```python
from build123d import *

# Parameters (mm, degrees)
SKETCH2_R           = 1.75
BOSS_EXTRUDE1_DEPTH = 10
SKETCH3_W           = 7.5
SKETCH3_H           = 3
BOSS_EXTRUDE2_DEPTH = 5
SKETCH4_W           = 15
SKETCH4_H           = 2
BOSS_EXTRUDE3_DEPTH = 20
SKETCH5_W           = 12
SKETCH5_H           = 17
CUT_EXTRUDE1_DEPTH  = 1
CUT_EXTRUDE2_DEPTH  = 12
BOSS_EXTRUDE4_DEPTH = 10
SKETCH8_W           = 7.5
SKETCH8_H           = 2
BOSS_EXTRUDE5_DEPTH = 11
BOSS_EXTRUDE6_START = -7.5
SKETCH9_R           = 2
BOSS_EXTRUDE6_DEPTH = 7.5
SKETCH10_R          = 1
CUT_EXTRUDE3_DEPTH  = 31.340772897


with BuildPart() as part:
    # Sketch2 → Boss-Extrude1 (new body)
    with BuildSketch(Plane(origin=(0, 0, 0), x_dir=(0, 0, -1), z_dir=(1, 0, 0))):
        Circle(SKETCH2_R)
    extrude(amount=BOSS_EXTRUDE1_DEPTH)

    # Sketch3 → Boss-Extrude2 (add)
    with BuildSketch(Plane.XY):
        with Locations((5, 0)):
            Rectangle(SKETCH3_W, SKETCH3_H)
    extrude(amount=BOSS_EXTRUDE2_DEPTH)

    # Sketch4 → Boss-Extrude3 (add)
    with BuildSketch(Plane.XY.offset(5)):
        with Locations((5, -0.5)):
            Rectangle(SKETCH4_W, SKETCH4_H)
    extrude(amount=BOSS_EXTRUDE3_DEPTH)

    # Sketch5 → Cut-Extrude1 (cut)
    with BuildSketch(Plane(origin=(0, 0.5, 0), x_dir=(1, 0, 0), z_dir=(0, 1, 0))):
        with Locations((5, -15)):
            Rectangle(SKETCH5_W, SKETCH5_H)
    extrude(amount=-CUT_EXTRUDE1_DEPTH, mode=Mode.SUBTRACT)

    # Sketch6 → Cut-Extrude2 (cut)
    with BuildSketch(Plane.ZY.offset(-11)):
        Polygon((23.5, -0.5), (25, 0.5), (23.5, 0.5), align=None)
    extrude(amount=CUT_EXTRUDE2_DEPTH, mode=Mode.SUBTRACT)

    # Sketch7 → Boss-Extrude4 (add)
    with BuildSketch(Plane(origin=(0, 0.5, 0), x_dir=(1, 0, 0), z_dir=(0, 1, 0))):
        Polygon((-2.5, -5), (12.5, -5), (12.5, -8), (11, -8), (11, -6.5), (-1, -6.5), (-1, -8), (-2.5, -8), align=None)
    extrude(amount=BOSS_EXTRUDE4_DEPTH)

    # Sketch8 → Boss-Extrude5 (add)
    with BuildSketch(Plane(origin=(0, 0, 0), x_dir=(1, 0, 0), z_dir=(0, 1, 0))):
        with Locations((5, 0.098612181)):
            Rectangle(SKETCH8_W, SKETCH8_H)
    extrude(amount=BOSS_EXTRUDE5_DEPTH)

    # Sketch9 → Boss-Extrude6 (add)
    with BuildSketch(Plane.ZY.offset(-1.25).offset(BOSS_EXTRUDE6_START)):
        with Locations((-0.098612181, 11)):
            Circle(SKETCH9_R)
    extrude(amount=BOSS_EXTRUDE6_DEPTH)

    # Sketch10 → Cut-Extrude3 (cut, through all)
    with BuildSketch(Plane.ZY.offset(-1.25)):
        with Locations((-0.098612181, 11)):
            Circle(SKETCH10_R)
    extrude(amount=-CUT_EXTRUDE3_DEPTH, mode=Mode.SUBTRACT)


solid = part.part
```
For this review, take the finished solid that the model builds, in its own axes (mm). A direction names the side the tool comes from. Coordinates: 2 decimals unless noted, no trailing zeros. Order: outer loops, then holes, each group sorted by start corner. A loop starts at its lowest first (then second) coordinate and runs counter-clockwise, first axis right, second up. Notation, with made-up numbers: (72.5, 71) -> (82.5, 71) arc R24 ccw to (82.5, 106) -> close; hole circle Ø9 at (48, 17.5). An arc over 180 degrees is marked (long way). Use CSV: the item, a comma, the result in double quotes. Start each with the question number.
Item 1: We need section A-A, the plane y = 8. Give the boundary of the cut face in (x, z), then the cut area to 3 significant figures.
Item 2: We need section B-B, the plane z = 8.75. Give the boundary of the cut face in (x, y), then the cut area to 3 significant figures.
Item 3: Wall thickness on probe 1 along X at (y, z) = (-0.25, 21); probe 2 along Z at (x, y) = (1.5, 1.75); probe 3 along X at (y, z) = (4, 0.5): over which ranges is each line inside the solid? List them lowest first.
Item 4: We need section D-D, the plane z = 0. Give the boundary of the cut face in (x, y), then the cut area to 3 significant figures.
Item 5: Draft analysis for pull direction X (two halves, no side actions). For faces 1 (the face through (5.084, -0.007, 24.24)), 2 (the face through (8.75, 7, 0)), 3 (the face through (0, 0, 0)), state which applies: pulls with the +X half, pulls with the -X half, needs draft (parallel to the pull), parting line crosses it, or undercut.
Item 6: Insertion check: pin 1 (0.8 mm diameter, centred on x = 12, y = 4.5, fed in from +Z); pin 2 (4.5 mm diameter, centred on y = 8.5, z = -0.5, fed in from +X); pin 3 (4 mm diameter, centred on y = 2, z = 2.5, fed in from -X); pin 4 (3.5 mm diameter, centred on y = 3, z = 19, fed in from -X). Each pin has a flat end and moves straight along its axis. Give the tip position at first contact, or say it passes through.
Item 7: For faces 4 (the face through (5, 5, -1.099)), 5 (the face through (11, 0, 12)), 6 (the face through (12, 0.5, 16)), list the 3-axis set-ups (+Z, -Z, +X, -X, +Y, -Y) from which the entire face can be reached by the end or side of a thin tool; tool diameter is ignored.
Item 8: We need section C-C, the plane x = 3. Give the boundary of the cut face in (y, z), then the cut area to 3 significant figures.
Derived:
1,outline,"(-2.5, 5) -> (12.5, 5) -> (12.5, 8) -> (11, 8) -> (11, 6.5) -> (-1, 6.5) -> (-1, 8) -> (-2.5, 8) -> close; (1.25, -1.1) -> (8.75, -1.1) -> (8.75, 0.9) -> (1.25, 0.9) -> close"
1,area,"42.0 mm^2"
2,outline,"(-2.5, -1.5) -> (12.5, -1.5) -> (12.5, 0.5) -> (11, 0.5) -> (11, -0.5) -> (-1, -0.5) -> (-1, 0.5) -> (-2.5, 0.5) -> close"
2,area,"18.0 mm^2"
3,probe 1,"x = -2.5 to -1, 11 to 12.5"
3,probe 2,"z = -1.1 to 0.9, 5 to 6.5"
3,probe 3,"x = 1.25 to 8.75"
4,outline,"(0, -1.75) -> (10, -1.75) -> (10, 1.75) -> (8.75, 1.75) -> (8.75, 10) -> (1.25, 10) -> (1.25, 1.75) -> (0, 1.75) -> close; (1.25, 12) -> (8.75, 12) -> (8.75, 13) -> (1.25, 13) -> close"
4,area,"104 mm^2"
5,face 1,"undercut"
5,face 2,"pulls with the +X half"
5,face 3,"pulls with the -X half"
6,pin 1,"stops at z = 8"
6,pin 2,"stops at x = 8.75"
6,pin 3,"stops at x = 0"
6,pin 4,"passes through"
7,face 4,"-Z, +X, -X"
7,face 5,"+Y"
7,face 6,"+Z, +X, -X, +Y"
8,outline,"(-1.5, 0.9) arc R1.75 ccw to (1.36, -1.1) -> (9.27, -1.1) arc R2 ccw (long way) to (9.27, 0.9) -> (1.5, 0.9) -> (1.5, 5) -> (10.5, 5) -> (10.5, 6.5) -> (-0.5, 6.5) -> (-0.5, 23.5) -> (0.5, 25) -> (-1.5, 25) -> close; hole circle Ø2 at (11, -0.1)"
8,area,"81.7 mm^2"
